from build123d import *

# Parameters (mm, degrees)
SKETCH_1_W          = 60
SKETCH_1_H          = 30
SKETCH_1_R          = 2
EXTRUDE_1_DEPTH     = 20
SKETCH_2_W          = 10
SKETCH_2_H          = 15
CUT_EXTRUDE_1_DEPTH = 47.904157598
SKETCH_3_R          = 7.5
CUT_EXTRUDE_2_DEPTH = 20
SKETCH_4_R          = 2
CUT_EXTRUDE_3_DEPTH = 47.904157598


with BuildPart() as part:
    # 스케치1 → 보스-돌출1 (new body)
    with BuildSketch(Plane(origin=(0, 0, 0), x_dir=(0, 0, -1), z_dir=(1, 0, 0))):
        Rectangle(SKETCH_1_W, SKETCH_1_H)
        with Locations((-23, 8)):
            Circle(SKETCH_1_R, mode=Mode.SUBTRACT)
        with Locations(Location((-23, -8, 0), (0, 0, 180))):
            Circle(SKETCH_1_R, mode=Mode.SUBTRACT)
        with Locations((23, -8)):
            Circle(SKETCH_1_R, mode=Mode.SUBTRACT)
        with Locations(Location((23, 8, 0), (0, 0, 180))):
            Circle(SKETCH_1_R, mode=Mode.SUBTRACT)
    extrude(amount=EXTRUDE_1_DEPTH)

    # 스케치2 → 컷-돌출1 (cut, through all)
    with BuildSketch(Plane(origin=(0, 15, 0), x_dir=(1, 0, 0), z_dir=(0, 1, 0))):
        with Locations((10, 22.5)):
            Rectangle(SKETCH_2_W, SKETCH_2_H)
        with Locations((10, -22.5)):
            Rectangle(SKETCH_2_W, SKETCH_2_H)
    extrude(amount=-CUT_EXTRUDE_1_DEPTH, mode=Mode.SUBTRACT)

    # 스케치3 → 컷-돌출2 (cut)
    with BuildSketch(Plane.ZY):
        Circle(SKETCH_3_R)
    extrude(amount=-CUT_EXTRUDE_2_DEPTH, mode=Mode.SUBTRACT)

    # 스케치4 → 컷-돌출3 (cut, through all)
    with BuildSketch(Plane(origin=(0, 15, 0), x_dir=(1, 0, 0), z_dir=(0, 1, 0))):
        with Locations(Location((10, 0, 0), (0, 0, 270))):
            Circle(SKETCH_4_R)
    extrude(amount=-CUT_EXTRUDE_3_DEPTH, mode=Mode.SUBTRACT)


solid = part.part
Work out the finished part from the listing and answer in its coordinate system (mm). A direction names the side the tool comes from. Give positions to 0.01 mm unless a question says otherwise; leave off trailing zeros. Order: outer loops, then holes, each group sorted by start corner. A loop starts at its lowest first (then second) coordinate and runs counter-clockwise, first axis right, second up. Notation, with made-up numbers: M -34.5,15.5 L -16.5,15.5 A15 ccw -16.5,32.5 Z; hole C -14,11.25 d9. An arc over 180 degrees is marked long. Return JSON: item names as keys, results as strings.
Q1. Find section B-B, the plane y = 0. Write down the section's boundary in (x, z), and give its area (3 significant figures).
Answer below:
{"outline": "M 0,-30 L 5,-30 L 5,-15 L 15,-15 L 15,-30 L 20,-30 L 20,-7.5 L 0,-7.5 Z; M 0,7.5 L 20,7.5 L 20,30 L 15,30 L 15,15 L 5,15 L 5,30 L 0,30 Z", "area": "600 mm^2"}
Q2. Which of the six approach directions +Z, -Z, +X, -X, +Y, -Y give full straight-line access (tool end or side, diameter ignored) to faces 4 (the face through (5, 0, -22)), 5 (the face through (10, 0, 15)), 6 (the face through (2.465, 6.648, -24.474))?
Answer below:
{"face 4": "-Z, +Y, -Y", "face 5": "+Z, +Y, -Y", "face 6": "+X, -X"}
Q3. Find section A-A, the plane x = 10. Write down the section's boundary in (y, z).
Answer below:
{"outline": "M -15,-15 L 15,-15 L 15,-2 L 7.23,-2 A7.5 cw -7.23,-2 L -15,-2 Z; M -15,2 L -7.23,2 A7.5 cw 7.23,2 L 15,2 L 15,15 L -15,15 Z"}
Q4. Find section D-D, the plane x = 18.5. Write down the section's boundary in (y, z), and give its area (3 significant figures).
Answer below:
{"outline": "M -15,-30 L 15,-30 L 15,30 L -15,30 Z; hole C -8,-23 d4; hole C -8,23 d4; hole C 0,0 d15; hole C 8,-23 d4; hole C 8,23 d4", "area": "1,570 mm^2"}
Q5. Find the intervals of material crossed by line 1 along Y through (x, z) = (2.1, -23); line 2 along Z through (x, y) = (2.65, 8); line 3 along Y through (x, z) = (6, -4.5), in increasing order. Write a range as [from, to].
Answer below:
{"line 1": "y = [-15, -10], [-6, 6], [10, 15]", "line 2": "z = [-30, -25], [-21, 21], [25, 30]", "line 3": "y = [-15, -6], [6, 15]"}
Q6. This flat-tipped pin is pushed along its axis until it touches: pin 1 (6 mm diameter, centred on x = 10.5, y = -5, fed in from -Z). Where does it stop, or does it pass through?
Answer below:
{"pin 1": "stops at z = -15"}
Q7. Find section C-C, the plane z = -23. Write down the section's boundary in (x, y), and give its area (3 significant figures).
Answer below:
{"outline": "M 0,-15 L 5,-15 L 5,-10 L 0,-10 Z; M 0,-6 L 5,-6 L 5,6 L 0,6 Z; M 0,10 L 5,10 L 5,15 L 0,15 Z; M 15,-15 L 20,-15 L 20,-10 L 15,-10 Z; M 15,-6 L 20,-6 L 20,6 L 15,6 Z; M 15,10 L 20,10 L 20,15 L 15,15 Z", "area": "220 mm^2"}
Q8. The mould has two halves that part along Y. Classify faces 1 (the face through (2, 0, -30)), 2 (the face through (7.6, -15, 0.4)), 3 (the face through (17, -8, -21)): pulls with the +Y half, pulls with the -Y half, needs draft (parallel to the pull), parting line crosses it, or undercut.
Answer below:
{"face 1": "needs draft", "face 2": "pulls with the -Y half", "face 3": "undercut"}
